Geometry: final body of the model. Coordinates: model frame, mm. A direction names the side the tool comes from. Give positions to 0.01 mm unless a question says otherwise; leave off trailing zeros. Write each loop counter-clockwise with the first axis right and the second up, starting at its lowest first coordinate (ties: lowest second). Pieces come first, ordered by that corner, then holes. Notation, with made-up numbers: M 28,19.5 L 61,19.5 A22 ccw 61,41.5 Z; hole C 15,58.5 d11. An arc over 180 degrees is marked long. Use a Markdown table: item, result. Add a question column.
(1) Pin query (flat end, axial travel): pin 1 Ø3.5 at (x, z) = (-35.5, -1.5) entering from +Y; pin 2 Ø8.5 at (x, z) = (37.5, 0) entering from -Y; pin 3 Ø12 at (y, z) = (25, -8) entering from -X; pin 4 Ø3 at (y, z) = (64, -2) entering from +X. Return the tip coordinate at first contact, or that it passes through.
(2) Draft query along X for faces 5 (the flat face through (41, 4, 0)), 6 (the flat face through (1, 0, 0)), 7 (the cylindrical face through (-43, 7, 0)), 8 (the flat face through (15, 29, 0)). Return one class per face: released by +X, released by -X, zero draft, split by the parting line, or undercut.
(3) Cut plane B-B (y = 63). Output: boundary loops of the cut face in (x, z), plus the area to 4 significant figures.
(4) Cut plane C-C (x = -37.5). Output: boundary loops of the cut face in (y, z).
(5) Reachability of faces 1 (the flat face through (31.8, 10, 0.1)), 2 (the cylindrical face through (32, 7, 0)), 3 (the flat face through (-43.2, 10, 0.1)), 4 (the flat face through (2.2, 74.2, 1)) from +Z, -Z, +X, -X, +Y, -Y: full face, straight path, thin tool, end or side. Return the list, or none.
(6) Cut plane D-D (y = 50). Output: boundary loops of the cut face in (x, z), plus the area to 3 significant figures.
(7) Material intervals for L1, parallel to Z at x = 37.5, y = 3.05; L2, parallel to Y at x = 0, z = 6.5; L3, parallel to Y at x = 36, z = 6.25, sorted ascending.
(8) Cut plane A-A (x = 0). Output: boundary loops of the cut face in (y, z).
```python
from build123d import *

# Parameters (mm, degrees)
SKETCH1_R                      = 15
BOSS_EXTRUDE1_DEPTH            = 10
SKETCH2_R                      = 15
SKETCH2_R_2                    = 6.25
BOSS_EXTRUDE2_DEPTH            = 10
FILLET1_R                      = 10
CBORE_FOR_M6_SHCS1_D           = 6.6
CBORE_FOR_M6_SHCS1_CBORE_D     = 11
CBORE_FOR_M6_SHCS1_CBORE_DEPTH = 6
SKETCH5_R                      = 15
SKETCH5_R_2                    = 11.25
BOSS_EXTRUDE3_DEPTH            = 1


with BuildPart() as part:
    # Sketch1 → Boss-Extrude1 (new, symmetric)
    with BuildSketch(Plane.XY):
        with BuildLine():
            Line((15, 43), (15, 10))
            Line((15, 10), (50, 10))
            Line((50, 10), (50, 0))
            Line((50, 0), (-50, 0))
            Line((-50, 0), (-50, 10))
            Line((-50, 10), (-15, 10))
            Line((-15, 10), (-15, 43))
            ThreePointArc((-15, 43), (0, 88), (15, 43))
        make_face()
        with Locations((0, 63)):
            Circle(SKETCH1_R, mode=Mode.SUBTRACT)
    extrude(amount=BOSS_EXTRUDE1_DEPTH, both=True)

    # Sketch2 → Boss-Extrude2 (add, through all)
    with BuildSketch(Plane.XY):
        with Locations((0, 63)):
            Circle(SKETCH2_R)
        with Locations((0, 63)):
            Circle(SKETCH2_R_2, mode=Mode.SUBTRACT)
    extrude(amount=-BOSS_EXTRUDE2_DEPTH)

    # Fillet1
    fillet1_edges = [part.edges().sort_by_distance(p)[0] for p in [
        (-15, 10, 0),
        (-15, 43, 0),
        (15, 43, 0),
        (15, 10, 0),
    ]]
    fillet(fillet1_edges, radius=FILLET1_R)

    # CBORE for M6 SHCS1 (through all)
    with Locations(Plane(origin=(0, 10, 0), x_dir=(1, 0, 0), z_dir=(0, 1, 0))):
        with Locations((-37.5, 0), (37.5, 0)):
            CounterBoreHole(CBORE_FOR_M6_SHCS1_D / 2, CBORE_FOR_M6_SHCS1_CBORE_D / 2, CBORE_FOR_M6_SHCS1_CBORE_DEPTH)

    # Sketch5 → Boss-Extrude3 (add)
    with BuildSketch(Plane.XY):
        with Locations((0, 63)):
            Circle(SKETCH5_R)
        with Locations((0, 63)):
            Circle(SKETCH5_R_2, mode=Mode.SUBTRACT)
    extrude(amount=BOSS_EXTRUDE3_DEPTH)


solid = part.part
```
Answer list:
| question | item | result |
|---|---|---|
| 1 | pin 1 | y = 4 |
| 1 | pin 2 | y = 0 |
| 1 | pin 3 | x = -15.05 |
| 1 | pin 4 | x = 25 |
| 2 | face 5 | undercut |
| 2 | face 6 | zero draft |
| 2 | face 7 | undercut |
| 2 | face 8 | released by +X |
| 3 | outline | M -25,-10 L -6.25,-10 L -6.25,0 L -11.25,0 L -11.25,1 L -15,1 L -15,10 L -25,10 Z; M 6.25,-10 L 25,-10 L 25,10 L 15,10 L 15,1 L 11.25,1 L 11.25,0 L 6.25,0 Z |
| 3 | area | 582.5 mm² |
| 4 | outline | M 0,-10 L 10,-10 L 10,-5.5 L 4,-5.5 L 4,-3.3 L 0,-3.3 Z; M 0,3.3 L 4,3.3 L 4,5.5 L 10,5.5 L 10,10 L 0,10 Z |
| 5 | face 1 | +Z, -Z, +X, +Y |
| 5 | face 2 | +Y |
| 5 | face 3 | +Z, -Z, -X, +Y |
| 5 | face 4 | +Z |
| 6 | outline | M -21.35,-10 L 21.35,-10 L 21.35,10 L 7.48,10 L 7.48,1 L -7.48,1 L -7.48,10 L -21.35,10 Z |
| 6 | area | 719 mm² |
| 7 | L1 | -10 to -3.3, 3.3 to 10 |
| 7 | L2 | 0 to 48, 78 to 88 |
| 7 | L3 | 0 to 10 |
| 8 | outline | M 0,-10 L 56.75,-10 L 56.75,0 L 51.75,0 L 51.75,1 L 48,1 L 48,10 L 0,10 Z; M 69.25,-10 L 88,-10 L 88,10 L 78,10 L 78,1 L 74.25,1 L 74.25,0 L 69.25,0 Z |
